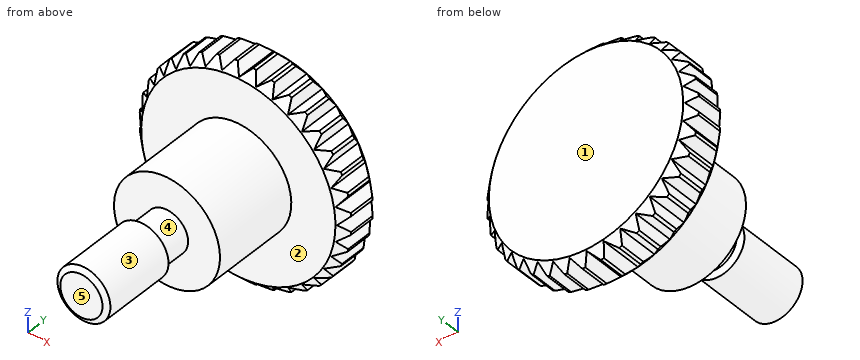
from build123d import *

# Parameters (mm, degrees)
POCKET_DEPTH       = 56.871497
POLARPATTERN_COUNT = 36


with BuildPart() as part:
    # Sketch → Revolution (revolve)
    with BuildSketch(Plane.YZ):
        Polygon((0, 0), (0, 1.195), (0.176092, 1.5), (4.25, 1.5), (4.426092, 1.195), (6, 1.195), (6, 3), (11, 3), (11, 5.5), (11.5, 6), (13, 6), (13.5, 5.5), (13.5, 0), align=None)
    revolve(axis=Axis((0, 0, 0), (0, 1, 0)))

    # Sketch001 → Pocket (cut, through all)
    with BuildSketch(Plane.ZX.offset(13.5)):
        Polygon((-0.5, 6.05), (0, 5.55), (0.5, 6.05), align=None)
    pocket = extrude(amount=-POCKET_DEPTH, mode=Mode.SUBTRACT)

    # PolarPattern: Pocket ×36 about axis
    polarpattern_axis = Axis((0, 13.5, 0), (0, 1, 0))
    for i in range(1, POLARPATTERN_COUNT):
        add(pocket.rotate(polarpattern_axis, i * 360 / POLARPATTERN_COUNT), mode=Mode.SUBTRACT)


solid = part.part
Build history of the part. All positions in model axes, mm. Face numbers are marked on the shaded views. A direction names the side the tool comes from. Coordinates: 2 decimals unless noted, no trailing zeros. Order: outer loops, then holes, each group sorted by start corner. A loop starts at its lowest first (then second) coordinate and runs counter-clockwise, first axis right, second up. Notation, with made-up numbers: (-3.75, 13) - (24.25, 13) arc R22 cw to (24.25, 46) - close; hole circle Ø10 at (52, 33.25). An arc over 180 degrees is marked (long way). Put each result on its own line as item: value.
1. Saw through at A-A (y = 2.25). Write the cut outline in (x, z), and give its area (3 significant figures).
Answer sheet:
outline: circle Ø3 at (0, 0)
area: 7.07 mm^2
2. Saw through at B-B (y = 6.5). Write the cut outline in (x, z), and give its area (3 significant figures).
Answer sheet:
outline: circle Ø6 at (0, 0)
area: 28.3 mm^2
3. Probe line 1 along X through (y, z) = (13.25, -1.5); line 2 along Y through (x, z) = (-2.25, -4.5); line 3 along X through (y, z) = (11.75, -0.5). List the from-to ranges inside material, lowest first. Write a range as [from, to].
Answer sheet:
line 1: x = [-5.55, 5.55]
line 2: y = [11, 13.5]
line 3: x = [-5.98, 5.98]
4. Pull direction Y, two halves, no side cores. Call the marked faces 3, 4 and 5: pulls with the +Y half, pulls with the -Y half, needs draft (parallel to the pull), parting line crosses it, or undercut.
Answer sheet:
face 3: needs draft
face 4: undercut
face 5: pulls with the -Y half
5. Tool access for the marked faces 1 and 2: list every direction of +Z, -Z, +X, -X, +Y, -Y with a clear straight run to the whole face (end or side of a thin tool).
Answer sheet:
face 1: +Z, -Z, +X, -X, +Y
face 2: -Y
6. Drop flat-ended pins along their axis: P1, Ø5, axis at y = 11, z = -3, coming from the -X side; P2, Ø1, axis at x = -2, z = -1.5, coming from the -Y side; P3, Ø6, axis at y = 7, z = -1, coming from the +X side. Give the stop position or say it passes through.
Answer sheet:
P1: stops at x = -5.97
P2: stops at y = 6
P3: stops at x = 3
